Drawing for the job (mm, zero at the part's lowest x, y, z). A direction names the side the tool comes from. Round coordinates to 2 decimals unless told otherwise and drop trailing zeros. Order: outer loops, then holes, each group sorted by start corner. A loop starts at its lowest first (then second) coordinate and runs counter-clockwise, first axis right, second up. Notation, with made-up numbers: (-36, -17.5) -> (-17, -17.5) arc R31 ccw to (-17, 8.5) -> close; hole circle Ø4 at (52, 3.25). An arc over 180 degrees is marked (long way). Use CSV: the item, a comma, the result in double quotes.
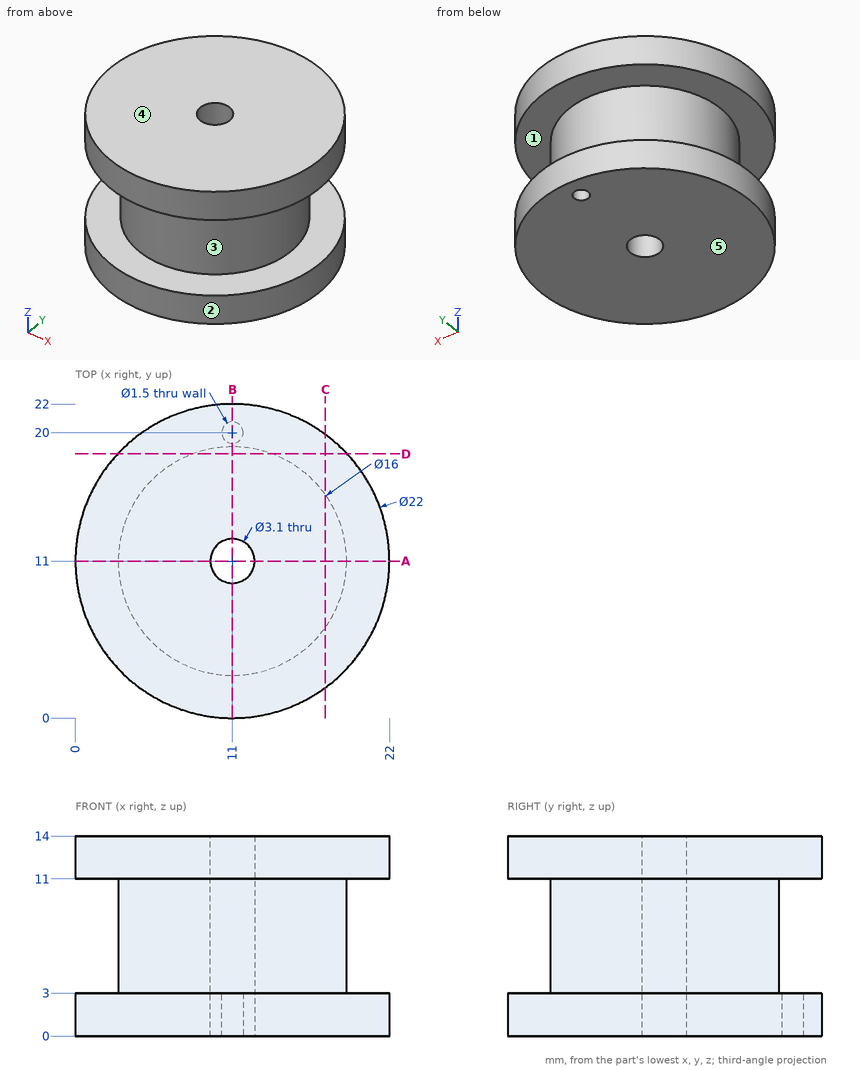
Q1. Which spindle directions (+Z, -Z, +X, -X, +Y, -Y) get a long thin tool onto all of the face, cutting with end or side? Do the marked faces 1 and 2. Say none if no direction does.
From the geometry:
face 1,"none"
face 2,"+Z, -Z"
Q2. Cut at B-B (x = 11). Give the cut face in (y, z), plus the area to 3 significant figures.
From the geometry:
outline,"(0, 0) -> (9.45, 0) -> (9.45, 14) -> (0, 14) -> (0, 11) -> (3, 11) -> (3, 3) -> (0, 3) -> close; (12.55, 0) -> (19.25, 0) -> (19.25, 3) -> (19, 3) -> (19, 11) -> (22, 11) -> (22, 14) -> (12.55, 14) -> close; (20.75, 0) -> (22, 0) -> (22, 3) -> (20.75, 3) -> close"
area,"212 mm²"
Q3. Probe line 1 along Y through (x, z) = (11, 2.25); line 2 along Z through (x, y) = (18.5, 19); line 3 along Y through (x, z) = (11, 8.25). List the from-to ranges inside material, lowest first.
From the geometry:
line 1,"y = 0 to 9.45, 12.55 to 19.25, 20.75 to 22"
line 2,"z = 0 to 3, 11 to 14"
line 3,"y = 3 to 9.45, 12.55 to 19"
Q4. Cut at D-D (y = 18.5). Give the cut face in (x, z).
From the geometry:
outline,"(2.95, 0) -> (19.05, 0) -> (19.05, 3) -> (13.78, 3) -> (13.78, 11) -> (19.05, 11) -> (19.05, 14) -> (2.95, 14) -> (2.95, 11) -> (8.22, 11) -> (8.22, 3) -> (2.95, 3) -> close"
Q5. Cut at A-A (y = 11). Give the cut face in (x, z), plus the area to 3 significant figures.
From the geometry:
outline,"(0, 0) -> (9.45, 0) -> (9.45, 14) -> (0, 14) -> (0, 11) -> (3, 11) -> (3, 3) -> (0, 3) -> close; (12.55, 0) -> (22, 0) -> (22, 3) -> (19, 3) -> (19, 11) -> (22, 11) -> (22, 14) -> (12.55, 14) -> close"
area,"217 mm²"
Q6. Pin check, flat tips, straight feed: pin 1 (8 mm diameter, centred on y = 3.5, z = 12.5, fed in from +X); pin 2 (4 mm diameter, centred on x = 3.5, z = 12.5, fed in from +Y); pin 3 (3 mm diameter, centred on y = 15.5, z = 9, fed in from +X). Stop position of each tip, or through.
From the geometry:
pin 1,"stops at x = 21.43"
pin 2,"stops at y = 20.53"
pin 3,"stops at x = 18.42"
Q7. Cut at C-C (x = 17.5). Give the cut face in (y, z), plus the area to 3 significant figures.
From the geometry:
outline,"(2.13, 0) -> (19.87, 0) -> (19.87, 3) -> (15.66, 3) -> (15.66, 11) -> (19.87, 11) -> (19.87, 14) -> (2.13, 14) -> (2.13, 11) -> (6.34, 11) -> (6.34, 3) -> (2.13, 3) -> close"
area,"181 mm²"
Q8. Mould opens along Z. For the marked faces 3, 4 and 5 say: +Z half, -Z half, draft (parallel to the pull), parting line (faces both ways), or undercut.
From the geometry:
face 3,"undercut"
face 4,"+Z half"
face 5,"-Z half"
